```python
from build123d import *

# Parameters (mm, degrees)
SKETCH_W     = 8
SKETCH_H     = 8
PAD_DEPTH    = 10
SKETCH001_R  = 2.291718
PAD001_DEPTH = 10


with BuildPart() as part:
    # Sketch → Pad (new body)
    with BuildSketch(Plane.YZ):
        Rectangle(SKETCH_W, SKETCH_H)
    extrude(amount=PAD_DEPTH)

    # Sketch001 (on Face6 of Pad) → Pad001 (join)
    with BuildSketch(Plane.YZ.offset(10)):
        Circle(SKETCH001_R)
    extrude(amount=PAD001_DEPTH)


solid = part.part
```
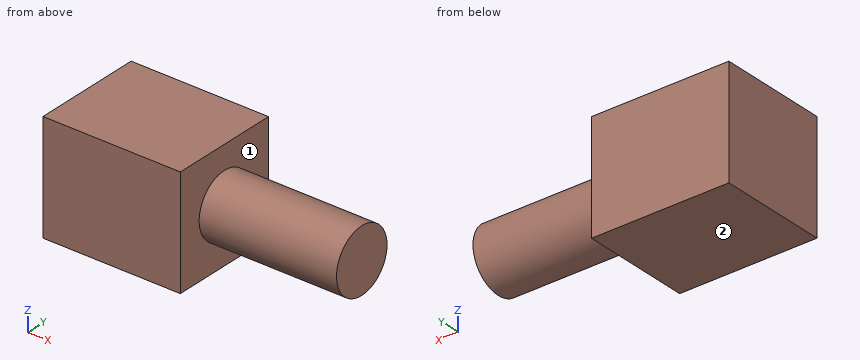
For this review, take the finished solid that the model builds, in its own axes (mm). Face numbers are marked on the shaded views. A direction names the side the tool comes from. Coordinates: 2 decimals unless noted, no trailing zeros. Write each loop counter-clockwise with the first axis right and the second up, starting at its lowest first coordinate (ties: lowest second). Pieces come first, ordered by that corner, then holes. Notation, with made-up numbers: (18.5, 34.25) -> (69.5, 34.25) arc R33 cw to (69.5, 63.25) -> close; hole circle Ø2 at (45, 89). An arc over 180 degrees is marked (long way). Put each result on its own line as item: value.
Q1. Tool access review of the marked faces 1 and 2: name each direction out of +Z, -Z, +X, -X, +Y, -Y from which nothing blocks a thin tool from reaching the whole face with its end or side.
From the geometry:
face 1: +X
face 2: -Z, +X, -X, +Y, -Y
Q2. Take a section at B-B, the plane z = -1. State the section outline as (x, y) points, then the cut area to 3 significant figures.
From the geometry:
outline: (0, -4) -> (10, -4) -> (10, -2.06) -> (20, -2.06) -> (20, 2.06) -> (10, 2.06) -> (10, 4) -> (0, 4) -> close
area: 121 mm2
Q3. Take a section at A-A, the plane y = 0. State the section outline as (x, z) points, then the cut area to 3 significant figures.
From the geometry:
outline: (0, -4) -> (10, -4) -> (10, -2.29) -> (20, -2.29) -> (20, 2.29) -> (10, 2.29) -> (10, 4) -> (0, 4) -> close
area: 126 mm2
Q4. Clearance check with flat-ended pins moving along their axes: pin 1 Ø3 at (x, y) = (16, 1.5) entering from +Z; pin 2 Ø1 at (y, z) = (-2, 2.5) entering from +X. State where each tip first meets the part, or that it passes through.
From the geometry:
pin 1: stops at z = 2.29
pin 2: stops at x = 10
Q5. Take a section at C-C, the plane y = 2.5. State the section outline as (x, z) points.
From the geometry:
outline: (0, -4) -> (10, -4) -> (10, 4) -> (0, 4) -> close
Q6. Wall thickness on L1, parallel to X at y = 2, z = 2.75; L2, parallel to Z at x = 12, y = -1.5; L3, parallel to Y at x = 10.5, z = -1: over which ranges is each line inside the solid? List them lowest first.
From the geometry:
L1: x = 0 to 10
L2: z = -1.73 to 1.73
L3: y = -2.06 to 2.06
